Input: part model. Units: mm. Frame: model coordinates. Coordinates: 2 decimals unless noted, no trailing zeros. Order: outer loops, then holes, each group sorted by start corner. A loop starts at its lowest first (then second) coordinate and runs counter-clockwise, first axis right, second up. Notation, with made-up numbers: (29.25, 64) - (47.25, 64) arc R24 cw to (47.25, 80) - close; hole circle Ø8 at (-31, 75.25). An arc over 180 degrees is marked (long way). Use a Markdown table: item, result. Add a question column.
from build123d import *

# Parameters (mm, degrees)
SKETCH1_W           = 473.075
SKETCH1_H           = 95.25
BOSS_EXTRUDE1_DEPTH = 3.175
SKETCH3_W           = 78.74
SKETCH3_H           = 51.308
CUT_EXTRUDE2_DEPTH  = 242.305221983
SKETCH4_R           = 8.255
CUT_EXTRUDE3_DEPTH  = 242.305221983
SKETCH5_R           = 1.5875
CUT_EXTRUDE4_DEPTH  = 242.305221983
SKETCH6_W           = 3.175
SKETCH6_H           = 95.25
BOSS_EXTRUDE2_DEPTH = 371.948016105
SKETCH7_R           = 3.81
SKETCH7_W           = 50.8
SKETCH7_H           = 73.025
CUT_EXTRUDE5_DEPTH  = 381
CUT_EXTRUDE6_DEPTH  = 381
SKETCH12_W          = 371.948016105
SKETCH12_H          = 95.25
CUT_EXTRUDE7_DEPTH  = 2.54
SKETCH14_W          = 473.075
SKETCH14_H          = 95.25
CUT_EXTRUDE8_DEPTH  = 3.175


with BuildPart() as part:
    # Sketch1 → Boss-Extrude1 (new body)
    with BuildSketch(Plane.XY):
        Rectangle(SKETCH1_W, SKETCH1_H)
    extrude(amount=BOSS_EXTRUDE1_DEPTH)

    # Sketch3 → Cut-Extrude2 (cut, through all)
    with BuildSketch(Plane.XY.offset(3.175)):
        with Locations((0, 6.731)):
            Rectangle(SKETCH3_W, SKETCH3_H)
    extrude(amount=-CUT_EXTRUDE2_DEPTH, mode=Mode.SUBTRACT)

    # Sketch4 → Cut-Extrude3 (cut, through all)
    with BuildSketch(Plane.XY.offset(3.175)):
        with Locations((37.592, -35.814)):
            Circle(SKETCH4_R)
    extrude(amount=-CUT_EXTRUDE3_DEPTH, mode=Mode.SUBTRACT)

    # Sketch5 → Cut-Extrude4 (cut, through all)
    with BuildSketch(Plane.XY.offset(3.175)):
        with Locations((-44.196, 40.259)):
            Circle(SKETCH5_R)
        with Locations((44.196, 40.259)):
            Circle(SKETCH5_R)
        with Locations((-44.196, -24.765)):
            Circle(SKETCH5_R)
        with Locations((44.196, -24.765)):
            Circle(SKETCH5_R)
    extrude(amount=-CUT_EXTRUDE4_DEPTH, mode=Mode.SUBTRACT)

    # Sketch6 → Boss-Extrude2 (add)
    with BuildSketch(Plane(origin=(0, 0, 0), x_dir=(-1, 0, 0), z_dir=(0, 0, -1))):
        with Locations((234.95, 0)):
            Rectangle(SKETCH6_W, SKETCH6_H)
    extrude(amount=BOSS_EXTRUDE2_DEPTH)

    # Sketch7 → Cut-Extrude5 (cut)
    with BuildSketch(Plane.ZY.offset(236.5375)):
        with Locations((-248.250016105, -28.575)):
            Circle(SKETCH7_R)
        with Locations((-308.448016105, -7.9375)):
            Rectangle(SKETCH7_W, SKETCH7_H)
    extrude(amount=-CUT_EXTRUDE5_DEPTH, mode=Mode.SUBTRACT)

    # Sketch8 → Cut-Extrude6 (cut)
    with BuildSketch(Plane.XY.offset(3.175)):
        with BuildLine():
            Line((88.9, 31.75), (215.9, 31.75))
            ThreePointArc((215.9, 31.75), (219.71, 27.94), (215.9, 24.13))
            Line((215.9, 24.13), (88.9, 24.13))
            ThreePointArc((88.9, 24.13), (85.09, 27.94), (88.9, 31.75))
        make_face()
        with BuildLine():
            Line((88.9, 12.563594852), (215.9, 12.563594852))
            ThreePointArc((215.9, 12.563594852), (219.71, 8.753594852), (215.9, 4.943594852))
            Line((215.9, 4.943594852), (88.9, 4.943594852))
            ThreePointArc((88.9, 4.943594852), (85.09, 8.753594852), (88.9, 12.563594852))
        make_face()
        with BuildLine():
            Line((88.9, -6.256272006), (215.9, -6.256272006))
            ThreePointArc((215.9, -6.256272006), (219.71, -10.066272006), (215.9, -13.876272006))
            Line((215.9, -13.876272006), (88.9, -13.876272006))
            ThreePointArc((88.9, -13.876272006), (85.09, -10.066272006), (88.9, -6.256272006))
        make_face()
        with BuildLine():
            Line((88.9, -24.84600572), (215.9, -24.84600572))
            ThreePointArc((215.9, -24.84600572), (219.71, -28.65600572), (215.9, -32.46600572))
            Line((215.9, -32.46600572), (88.9, -32.46600572))
            ThreePointArc((88.9, -32.46600572), (85.09, -28.65600572), (88.9, -24.84600572))
        make_face()
        with BuildLine():
            Line((-88.9, -24.84600572), (-215.9, -24.84600572))
            ThreePointArc((-215.9, -24.84600572), (-219.71, -28.65600572), (-215.9, -32.46600572))
            Line((-215.9, -32.46600572), (-88.9, -32.46600572))
            ThreePointArc((-88.9, -32.46600572), (-85.09, -28.65600572), (-88.9, -24.84600572))
        make_face()
        with BuildLine():
            Line((-88.9, -6.256272006), (-215.9, -6.256272006))
            ThreePointArc((-215.9, -6.256272006), (-219.71, -10.066272006), (-215.9, -13.876272006))
            Line((-215.9, -13.876272006), (-88.9, -13.876272006))
            ThreePointArc((-88.9, -13.876272006), (-85.09, -10.066272006), (-88.9, -6.256272006))
        make_face()
        with BuildLine():
            Line((-88.9, 12.563594852), (-215.9, 12.563594852))
            ThreePointArc((-215.9, 12.563594852), (-219.71, 8.753594852), (-215.9, 4.943594852))
            Line((-215.9, 4.943594852), (-88.9, 4.943594852))
            ThreePointArc((-88.9, 4.943594852), (-85.09, 8.753594852), (-88.9, 12.563594852))
        make_face()
        with BuildLine():
            Line((-88.9, 31.75), (-215.9, 31.75))
            ThreePointArc((-215.9, 31.75), (-219.71, 27.94), (-215.9, 24.13))
            Line((-215.9, 24.13), (-88.9, 24.13))
            ThreePointArc((-88.9, 24.13), (-85.09, 27.94), (-88.9, 31.75))
        make_face()
    extrude(amount=-CUT_EXTRUDE6_DEPTH, mode=Mode.SUBTRACT)

    # Sketch12 → Cut-Extrude7 (cut)
    with BuildSketch(Plane(origin=(-233.3625, 0, 0), x_dir=(0, 0, -1), z_dir=(1, 0, 0))):
        with Locations((185.974008053, 0)):
            Rectangle(SKETCH12_W, SKETCH12_H)
    extrude(amount=-CUT_EXTRUDE7_DEPTH, mode=Mode.SUBTRACT)

    # Sketch14 → Cut-Extrude8 (cut)
    with BuildSketch(Plane.XY.offset(3.175)):
        Rectangle(SKETCH14_W, SKETCH14_H)
    extrude(amount=-CUT_EXTRUDE8_DEPTH, mode=Mode.SUBTRACT)


solid = part.part
1) Cut plane C-C (x = -236.3). Return the cut outline in (y, z) (3 decimals), and give its area (3 significant figures).
2) Material intervals for L1, parallel to Z at x = -236.2, y = -40; L2, parallel to Y at x = -236.1, z = -300.5 (3 decimals), sorted ascending.
3) Cut plane A-A (y = -10). Return the cut outline in (x, z), and give its area (3 significant figures).
4) Pull-direction query (Y, two-part tool) for faces 1 (the cylindrical face through (-236.224, -27.431, -244.616)), 2 (the flat face through (-236.538, -1, -183)); classes: pulls with the +Y half, pulls with the -Y half, needs draft (parallel to the pull), parting line crosses it, or undercut.
Computed:
| question | item | result |
|---|---|---|
| 1 | outline | (-47.625, -371.948) - (47.625, -371.948) - (47.625, 0) - (-47.625, 0) - close; hole (-44.45, -333.848) - (28.575, -333.848) - (28.575, -283.048) - (-44.45, -283.048) - close; hole circle Ø7.62 at (-28.575, -248.25) |
| 1 | area | 31,700 mm2 |
| 2 | L1 | z = -371.95 to -333.85, -283.05 to 0 |
| 2 | L2 | y = -47.625 to -44.45, 28.575 to 47.625 |
| 3 | outline | (-236.54, -371.95) - (-235.9, -371.95) - (-235.9, -333.85) - (-236.54, -333.85) - close; (-236.54, -283.05) - (-235.9, -283.05) - (-235.9, 0) - (-236.54, 0) - close |
| 3 | area | 204 mm2 |
| 4 | face 1 | undercut |
| 4 | face 2 | needs draft |
